Input: part model. Units: mm. Frame: model coordinates. A direction names the side the tool comes from. Coordinates: 2 decimals unless noted, no trailing zeros. Order: outer loops, then holes, each group sorted by start corner. A loop starts at its lowest first (then second) coordinate and runs counter-clockwise, first axis right, second up. Notation, with made-up numbers: M 79.25,-3 L 135.25,-3 A18 ccw 135.25,21 Z; hole C 89,55 d5. An arc over 180 degrees is marked long. Answer in a Markdown table with one row per item.
from build123d import *

# Parameters (mm, degrees)
F0_R          = 52.07
F0_R_2        = 49.53
F4_DEPTH      = 50.8
F4_DEPTH_BACK = 50.8


with BuildPart() as f2:
    # F2: sweep along a path in F1
    with BuildLine(Plane.YZ) as f2_path:
        Line((0, 0), (0, 25.4))
        Line((0, 25.4), (-7.4446247891, 48.2820980251))
        Line((-7.4446247891, 48.2820980251), (-21.4247759432, 61.7959573865))
    # F0 (on Top) → F2 (sweep)
    with BuildSketch(Plane.XY):
        Circle(F0_R)
        Circle(F0_R_2, mode=Mode.SUBTRACT)
    sweep(path=f2_path.line, transition=Transition.RIGHT)

    # F3 (on Right) → F4 (cut, two sides)
    with BuildSketch(Plane.YZ) as f4_sk:
        with BuildLine():
            ThreePointArc((11.6053752109, 48.2820980251), (43.3553752109, 16.5320980251), (75.1053752109, 48.2820980251))
            ThreePointArc((75.1053752109, 48.2820980251), (43.3553752109, 80.0320980251), (11.6053752109, 48.2820980251))
        make_face()
    extrude(amount=-F4_DEPTH, mode=Mode.SUBTRACT)
    extrude(f4_sk.sketch, amount=F4_DEPTH_BACK, mode=Mode.SUBTRACT)


solid = f2.part
1) Reachability of faces 1 (the face through (46, -19, 0)), 2 (the face through (49.666, 15.64, 11.226)) from +Z, -Z, +X, -X, +Y, -Y: full face, straight path, thin tool, end or side. Return the list, or none.
Resolved:
| item | result |
|---|---|
| face 1 | -Z, +X, -X, +Y, -Y |
| face 2 | -Z |
2) Cut plane C-C, the plane y = 23.5. State how many separate pieces and enclosed holes the cut face has, and give its area (3 significant figures).
Resolved:
| item | result |
|---|---|
| separate pieces | 3 |
| enclosed holes | 0 |
| area | 381 mm2 |
3) Cut plane B-B, the plane x = 17. Output: boundary loops of the cut face in (y, z), and give its area (3 significant figures).
Resolved:
| item | result |
|---|---|
| outline | M -55.63,26.41 L -50.46,21.41 L -49.22,17.6 L -49.22,0 L -46.52,0 L -46.52,18.02 L -48.1,22.88 L -53.76,28.35 Z; M 10.91,95.24 L 29.79,76.99 A31.75 cw 32.5,78.12 L 12.78,97.18 Z; M 46.52,0 L 49.22,0 L 49.22,17.08 A31.75 cw 46.52,16.69 Z |
| area | 198 mm2 |
4) Cut plane A-A, the plane x = -18. Output: boundary loops of the cut face in (y, z).
Resolved:
| item | result |
|---|---|
| outline | M -55.38,26.67 L -50.15,21.6 L -48.86,17.65 L -48.86,0 L -46.14,0 L -46.14,18.08 L -47.77,23.09 L -53.5,28.62 Z; M 10.65,94.97 L 29.43,76.82 A31.75 cw 32.13,77.98 L 12.53,96.93 Z; M 46.14,0 L 48.86,0 L 48.86,17.01 A31.75 cw 46.14,16.65 Z |
5) Mould query, pull axis X, two halves, no side actions, for faces 3 (the face through (-24.59, -46.82, 20.95)), 4 (the face through (45.753, -18.97, 11.226)), 5 (the face through (-19.042, -53.424, 28.692)). Classes: +X half, -X half, draft (parallel to the pull), parting line (faces both ways), or undercut.
Resolved:
| item | result |
|---|---|
| face 3 | parting line |
| face 4 | undercut |
| face 5 | draft |
6) Material intervals for probe 1 along Y at (x, z) = (0, 8); probe 2 along X at (y, z) = (9.5, 26); probe 3 along Y at (x, z) = (-41, 6.5), sorted ascending.
Resolved:
| item | result |
|---|---|
| probe 1 | y = -52.07 to -49.53, 49.53 to 52.07 |
| probe 2 | x = -51.2 to -48.61, 48.61 to 51.2 |
| probe 3 | y = -32.1 to -27.79, 27.79 to 32.1 |
7) Contact query for flat-ended pins moving along their axis: pin 1 (6 mm diameter, centred on y = -27.5, z = 28, fed in from +X); pin 2 (6 mm diameter, centred on y = 4, z = 66, fed in from +X); pin 3 (10 mm diameter, centred on x = 35, y = 9.5, fed in from -Z); pin 4 (3 mm diameter, centred on y = 17, z = 59, fed in from -X). Output: stop coordinate, or through.
Resolved:
| item | result |
|---|---|
| pin 1 | stops at x = 47.03 |
| pin 2 | stops at x = 48.97 |
| pin 3 | stops at z = 71.35 |
| pin 4 | passes through |
